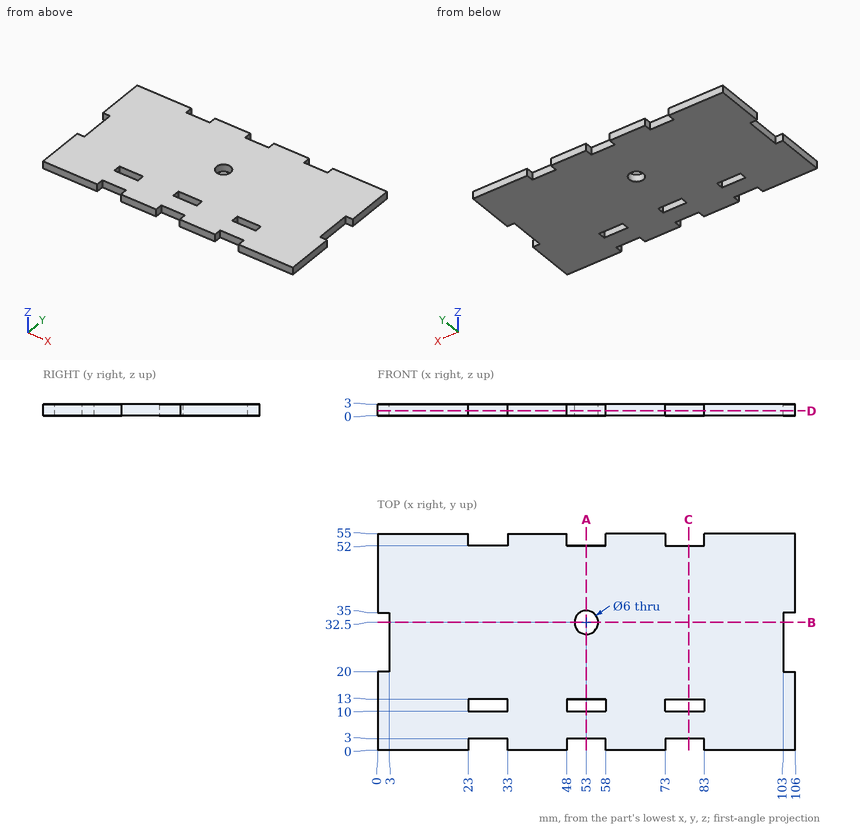
Job drawing, mm, ordinate dimensions from the low corner. One solid piece. Round coordinates to 2 decimals unless told otherwise and drop trailing zeros. Loops run counter-clockwise (first coordinate to the right, second up) from the corner with the lowest first, then second, coordinate; pieces in that order, holes last. Notation, with made-up numbers: (62.25, -20.5) -> (117.25, -20.5) arc R22 ccw to (117.25, 18.5) -> close; hole circle Ø4 at (47.25, -32.5). An arc over 180 degrees is marked (long way). One line per item, written item: value. Start each with the question number.
Q1. Drop flat-ended pins along their axis: pin 1 Ø8 at (x, y) = (53, 32.5) entering from -Z; pin 2 Ø1.5 at (x, z) = (54.5, 2) entering from +Y; pin 3 Ø1.5 at (x, z) = (50.5, 2) entering from -Y. Give the stop position or say it passes through.
Q2. Cut at A-A on x = 53. List the corners of the cut face in (y, z).
Q3. Cut at D-D on z = 1.25. Count the separate pieces of the cut face and the enclosed holes in it, plus the area to 3 significant figures.
Q4. Cut at C-C on x = 79. List the corners of the cut face in (y, z), plus the area to 3 significant figures.
Q5. Probe line 1 along X through (y, z) = (11, 2.5); line 2 along Y through (x, z) = (53, 0.95); line 3 along Y through (x, z) = (55.5, 1.55). List the from-to ranges inside material, lowest first.
Q6. Cut at B-B on y = 32.5. List the corners of the cut face in (x, z).
Computed:
1. pin 1: z = 0
1. pin 2: y = 52
1. pin 3: y = 3
2. outline: (3, 0) -> (10, 0) -> (10, 3) -> (3, 3) -> close; (13, 0) -> (29.5, 0) -> (29.5, 3) -> (13, 3) -> close; (35.5, 0) -> (52, 0) -> (52, 3) -> (35.5, 3) -> close
3. separate pieces: 1
3. enclosed holes: 4
3. area: 5,440 mm²
4. outline: (3, 0) -> (10, 0) -> (10, 3) -> (3, 3) -> close; (13, 0) -> (52, 0) -> (52, 3) -> (13, 3) -> close
4. area: 138 mm²
5. line 1: 0 to 23, 33 to 48, 58 to 73, 83 to 106
5. line 2: 3 to 10, 13 to 29.5, 35.5 to 52
5. line 3: 3 to 10, 13 to 30.84, 34.16 to 52
6. outline: (3, 0) -> (50, 0) -> (50, 3) -> (3, 3) -> close; (56, 0) -> (103, 0) -> (103, 3) -> (56, 3) -> close
